Part model, mm, in its own coordinate system. A direction names the side the tool comes from. Round coordinates to 2 decimals unless told otherwise and drop trailing zeros. Write each loop counter-clockwise with the first axis right and the second up, starting at its lowest first coordinate (ties: lowest second). Pieces come first, ordered by that corner, then holes.
```python
from build123d import *

# Parameters (mm, degrees)
SKETCH1_R           = 3.125
BOSS_EXTRUDE1_DEPTH = 8
SKETCH2_W           = 2.25
SKETCH2_H           = 3.25
CUT_EXTRUDE1_DEPTH  = 3
FILLET1_R           = 1


with BuildPart() as part:
    # Sketch1 → Boss-Extrude1 (new body)
    with BuildSketch(Plane(origin=(0, 0, 0), x_dir=(1, 0, 0), z_dir=(0, 1, 0))):
        Circle(SKETCH1_R)
    extrude(amount=BOSS_EXTRUDE1_DEPTH)

    # Sketch2 → Cut-Extrude1 (cut)
    with BuildSketch(Plane.XZ):
        Rectangle(SKETCH2_W, SKETCH2_H)
    extrude(amount=-CUT_EXTRUDE1_DEPTH, mode=Mode.SUBTRACT)

    # Fillet1
    fillet1_edges = [part.edges().sort_by_distance(p)[0] for p in [
        (-3.125, 8, 0),
    ]]
    fillet(fillet1_edges, radius=FILLET1_R)


solid = part.part
```
Q1. Cut at B-B on x = 0. Write the cut outline in (y, z) (3 decimals), plus the area to 3 significant figures.
Values follow:
outline: (0, -3.125) - (7, -3.125) arc R1 ccw to (8, -2.125) - (8, 2.125) arc R1 ccw to (7, 3.125) - (0, 3.125) - (0, 1.625) - (3, 1.625) - (3, -1.625) - (0, -1.625) - close
area: 39.8 mm2
Q2. Mould opens along Z. For faces 3 (the cylindrical face through (2.98, 3.45, -0.94)), 4 (the flat face through (1.3, 0, 0)), 5 (the flat face through (1.125, 1, 0)) say: +Z half, -Z half, draft (parallel to the pull), parting line (faces both ways), or undercut.
Values follow:
face 3: parting line
face 4: draft
face 5: undercut
Q3. Wall check: L1, parallel to Y at x = -0.75, z = -0.5; L2, parallel to X at y = 1.5, z = -1.5 (3 decimals); L3, parallel to Z at x = 0.75, y = 1 (3 decimals). Give the ranges that are in metal, low to high.
Values follow:
L1: y = 3 to 8
L2: x = -2.741 to -1.125, 1.125 to 2.741
L3: z = -3.034 to -1.625, 1.625 to 3.034
Q4. Which spindle directions (+Z, -Z, +X, -X, +Y, -Y) get a long thin tool onto all of the face, cutting with end or side? Do faces 1 (the flat face through (0, 8, 0)), 2 (the flat face through (0, 1, -1.625)). Say none if no direction does.
Values follow:
face 1: +Z, -Z, +X, -X, +Y
face 2: -Y
Q5. Cut at A-A on y = 1.25. Write the cut outline in (x, z) (3 decimals), plus the area to 3 significant figures.
Values follow:
outline: circle Ø6.25 at (0, 0); hole (-1.125, -1.625) - (1.125, -1.625) - (1.125, 1.625) - (-1.125, 1.625) - close
area: 23.4 mm2
Q6. Drop flat-ended pins along their axis: pin 1 (1 mm diameter, centred on y = 1.5, z = -1, fed in from +X); pin 2 (1 mm diameter, centred on y = 3.5, z = 1.5, fed in from +X); pin 3 (3 mm diameter, centred on y = 6.5, z = 1.5, fed in from -X) (3 decimals); pin 4 (0.7 mm diameter, centred on x = -0.5, z = 1, fed in from -Y). Give the stop position or say it passes through.
Values follow:
pin 1: stops at x = 3.08
pin 2: stops at x = 2.96
pin 3: stops at x = -3.125
pin 4: stops at y = 3
Q7. Cut at C-C on z = 0. Write the cut outline in (x, y) (3 decimals), plus the area to 3 significant figures.
Values follow:
outline: (-3.125, 0) - (-1.125, 0) - (-1.125, 3) - (1.125, 3) - (1.125, 0) - (3.125, 0) - (3.125, 7) arc R1 ccw to (2.125, 8) - (-2.125, 8) arc R1 ccw to (-3.125, 7) - close
area: 42.8 mm2
